Autodesk Inventor part; units mm, degrees
ref_plane "YZ Plane" through (0, 0, 0) normal (1, 0, 0) x (0, 1, 0)
ref_plane "XZ Plane" through (0, 0, 0) normal (0, 1, 0) x (-1, 0, 0)
ref_plane "XY Plane" through (0, 0, 0) normal (0, 0, 1) x (1, 0, 0)
sketch "Sketch1" plane through (0, 0, 0) normal (0, 1, 0) x (-1, 0, 0)
  line L0 (0, 0) -> (0, -21)
  line L1 (0, -21) -> (-43.6, -21)
  line L2 (-43.6, -21) -> (-43.6, 0)
  line L3 (-43.6, 0) -> (0, 0)
  line L4 (-43.6, 0) -> (-38.6, 0)
  circle A0 centre (-37, -2.5049) radius 1.5
  line L5 (0, -21) -> (-5, -21)
  circle A1 centre (-6.6, -18.5) radius 1.5
  dimension "d0" = 21
  dimension "d1" = 43.6
  dimension "d5" = 3
  dimension "d9" = 3
extrude "Extrusion1" add sketch "Sketch1" along normal blind 13.2
properties part number "boost_converter"
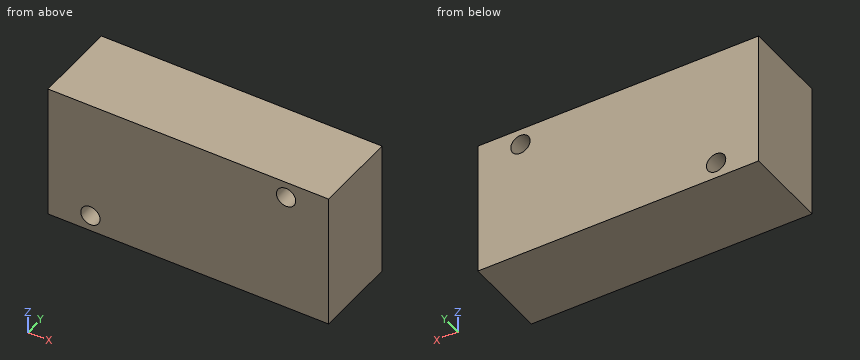
Work out the finished part from the listing and answer in its coordinate system (mm). Give positions to 0.01 mm unless a question says otherwise; leave off trailing zeros. Write each loop counter-clockwise with the first axis right and the second up, starting at its lowest first coordinate (ties: lowest second). Pieces come first, ordered by that corner, then holes. Notation, with made-up numbers: (-9, 21.5) - (36, 21.5) arc R30 cw to (36, 59.5) - close; hole circle Ø4 at (6, 68). An arc over 180 degrees is marked (long way). Use one line per item in the form item = value.
1. This flat-tipped pin is pushed along its axis until it touches: pin 1 Ø3 at (x, y) = (31, 6.5) entering from +Z. Where does it stop, or does it pass through?
Filled in:
pin_1 = 0
2. Consider L1, parallel to Z at x = 37, y = 9; L2, parallel to Z at x = 6.6, y = 4.75; L3, parallel to X at y = 1.5, z = -19. Determine where each line is inside the solid, lowest interval first.
Filled in:
L1 = -21 to -4, -1 to 0
L2 = -21 to -20, -17 to 0
L3 = 0 to 5.19, 8.01 to 43.6
3. A cutting plane is placed at A-A (x = 37). Write down the section's boundary in (y, z).
Filled in:
outline = (0, -21) - (13.2, -21) - (13.2, -4) - (0, -4) - close; (0, -1) - (13.2, -1) - (13.2, 0) - (0, 0) - close
4. A cutting plane is placed at B-B (z = -18.5). Write down the section's boundary in (x, y), and give its area (3 significant figures).
Filled in:
outline = (0, 0) - (5.1, 0) - (5.1, 13.2) - (0, 13.2) - close; (8.1, 0) - (43.6, 0) - (43.6, 13.2) - (8.1, 13.2) - close
area = 536 mm^2
5. A cutting plane is placed at C-C (y = 1.75). Write down the section's boundary in (x, z).
Filled in:
outline = (0, -21) - (43.6, -21) - (43.6, 0) - (0, 0) - close; hole circle Ø3 at (6.6, -18.5); hole circle Ø3 at (37, -2.5)
